Could you check a few things on this drawing? It's one solid part, dimensions in mm from its lowest x, y, z. A direction names the side the tool comes from. Coordinates: 2 decimals unless noted, no trailing zeros. Loops run counter-clockwise (first coordinate to the right, second up) from the corner with the lowest first, then second, coordinate; pieces in that order, holes last. Notation, with made-up numbers: M -27,-10 L -2,-10 A12 ccw -2,13 Z; hole C 85,3 d11. An arc over 180 degrees is marked long. Use one line per item in the form item = value. Start each with the question number.
(1) Will these pins go through, and if not, where does the flat tip stop? P1, Ø8, axis at y = 24.5, z = 4, coming from the +X side; P2, Ø6, axis at x = 11, z = 8.5, coming from the +Y side; P3, Ø4, axis at x = 67, z = 6.5, coming from the -Y side.
(2) Imagine slicing it at A-A, the plane y = 21. Please give me the cut outline in (x, z).
(3) Imagine slicing it at B-B, the plane x = 5. Please give me the cut outline in (y, z).
(4) Imagine slicing it at D-D, the plane y = 31.5. Please give me the cut outline in (x, z), and give its area (3 significant figures).
(5) On a 3-axis mill with a long thin cutter (end or side, diameter ignored), from which of +Z, -Z, +X, -X, +Y, -Y can I reach the whole of each face in a straight line? I mean the marked faces 1, 2, 3, 4 and 5. Say none if no direction works.
(6) Please list where these lines run through material, in increasing order: L1, parallel to X at y = 19.5, z = 2; L2, parallel to Y at x = 27, z = 21; L3, parallel to Y at x = 63.5, z = 18.5 (1 decimal).
(7) Imagine slicing it at C-C, the plane z = 9. Please give me the cut outline in (x, y), and give its area (3 significant figures).
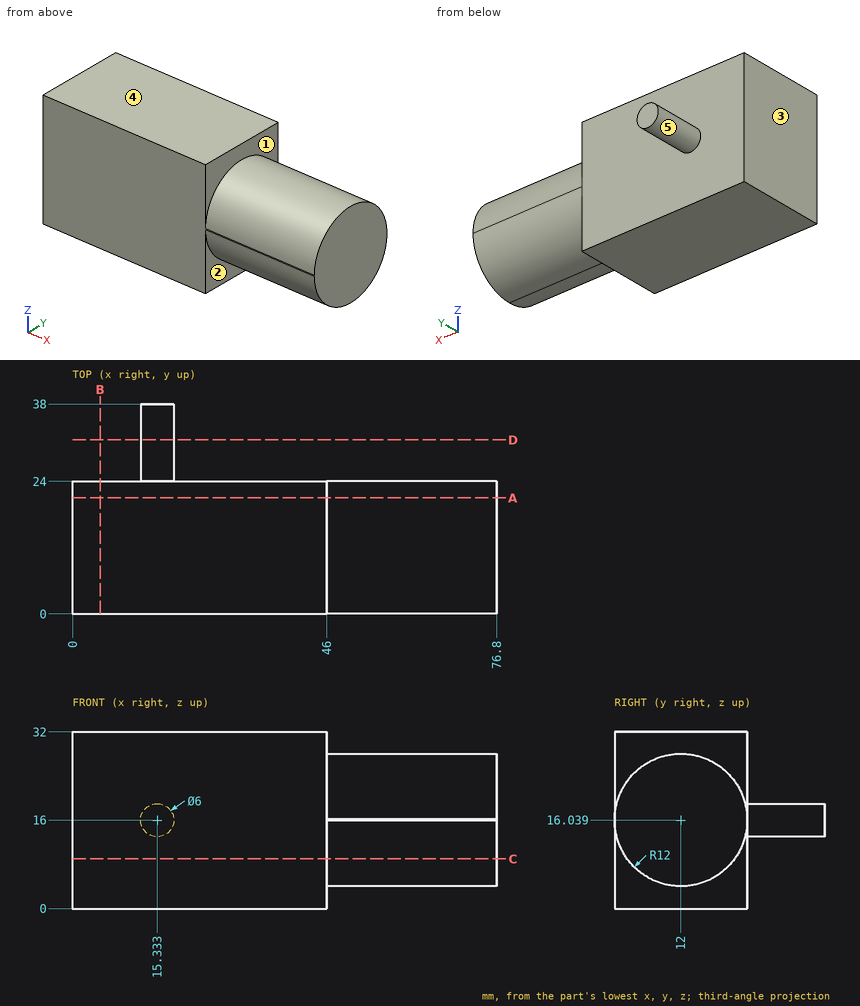
Answer:
q1.P1 = 46
q1.P2 = 24
q1.P3 = 2.66
q2.outline = M 0,0 L 46,0 L 46,8.1 L 76.8,8.1 L 76.8,23.98 L 46,23.98 L 46,32 L 0,32 Z
q3.outline = M 0,0 L 24,0 L 24,32 L 0,32 Z
q4.outline = C 15.33,16 d6
q4.area = 28.3 mm²
q5.face_1 = +Z, +X
q5.face_2 = -Z, +X
q5.face_3 = +Z, -Z, -X, +Y, -Y
q5.face_4 = +Z, +X, -X, +Y, -Y
q5.face_5 = +Y
q6.L1 = 0 to 46
q6.L2 = 0 to 24
q6.L3 = 0.3 to 23.7
q7.outline = M 0,0 L 46,0 L 46,2.28 L 76.8,2.28 L 76.8,21.72 L 46,21.72 L 46,24 L 0,24 Z
q7.area = 1,700 mm²
